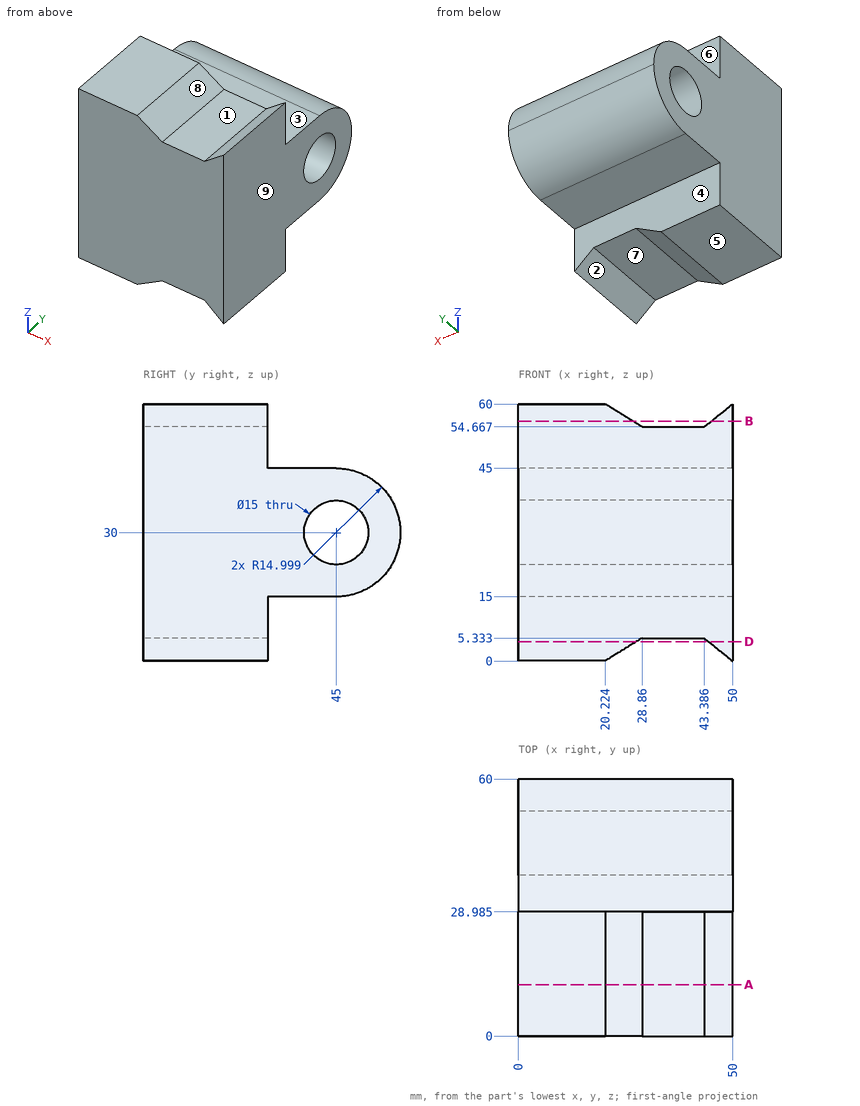
Design review of the part shown in the three views and the two pictorial views. Dimensions are in mm from the part's minimum x, y and z. A direction names the side the tool comes from. Round coordinates to 2 decimals unless told otherwise and drop trailing zeros. Write each loop counter-clockwise with the first axis right and the second up, starting at its lowest first coordinate (ties: lowest second). Pieces come first, ordered by that corner, then holes.
Item 1: For pin 1 Ø5 at (x, y) = (21, 33) entering from -Z; pin 2 Ø1.5 at (x, z) = (34, 26) entering from +Y; pin 3 Ø4.5 at (x, y) = (36.5, 9.5) entering from +Z, all flat-tipped, find the tip position at first contact; note any pin that passes through.
Item 2: Draft analysis for pull direction X (two halves, no side actions). For the marked faces 6, 7, 8 and 9, state which applies: released by +X, released by -X, zero draft, split by the parting line, or undercut.
Item 3: Wall thickness on L1, parallel to Y at x = 20.5, z = 30; L2, parallel to Z at x = 38.5, y = 44.5; L3, parallel to Y at x = 8, z = 6 (1 decimal): over which ranges is each line inside the solid? List them lowest first.
Item 4: Consider section A-A on y = 12. Give the boundary of the cut face in (x, z) (1 decimal), and give its area (3 significant figures).
Item 5: Consider section D-D on z = 4.5. Give the boundary of the cut face in (x, y) (1 decimal).
Item 6: For the marked faces 1, 2, 3, 4 and 5, list the 3-axis set-ups (+Z, -Z, +X, -X, +Y, -Y) from which the entire face can be reached by the end or side of a thin tool; tool diameter is ignored.
Item 7: Consider section B-B on z = 56. Give the boundary of the cut face in (x, y) (1 decimal).
Check values:
1. pin 1: stops at z = 15
1. pin 2: stops at y = 59.64
1. pin 3: stops at z = 54.67
2. face 6: zero draft
2. face 7: undercut
2. face 8: undercut
2. face 9: released by +X
3. L1: y = 0 to 37.5, 52.5 to 60
3. L2: z = 15 to 22.52, 37.48 to 45
3. L3: y = 0 to 29
4. outline: (0, 0) - (20.2, 0) - (28.9, 5.3) - (43.4, 5.3) - (50, 0) - (50, 60) - (43.4, 54.7) - (28.9, 54.7) - (20.2, 60) - (0, 60) - close
4. area: 2,760 mm2
5. outline: (0, 0) - (27.5, 0) - (27.5, 29) - (0, 29) - close; (44.4, 0) - (50, 0) - (50, 29) - (44.4, 29) - close
6. face 1: +Z, +Y, -Y
6. face 2: -Z, +Y, -Y
6. face 3: +Z, +X, -X, +Y
6. face 4: -Z, +X, -X, +Y
6. face 5: -Z, +X, -X, +Y, -Y
7. outline: (0, 0) - (26.7, 0) - (26.7, 29) - (0, 29) - close; (45, 0) - (50, 0) - (50, 29) - (45, 29) - close
